```python
from build123d import *

# Parameters (mm, degrees)
F0_W          = 50.5
F0_H          = 50.5
F1_DEPTH      = 7.2
F2_W          = 45.2
F2_H          = 45.2
F3_DEPTH      = 5
F4_W          = 42
F4_H          = 42
F5_DEPTH      = 5
F5_DEPTH_BACK = 3
F6_R          = 2.5
F7_R          = 2
F8_SIZE       = 1
F9_R          = 1


with BuildPart() as f1:
    # F0 (on Top) → F1 (new body)
    with BuildSketch(Plane.XY):
        Rectangle(F0_W, F0_H)
    extrude(amount=F1_DEPTH)

    # F2 (on face) → F3 (join)
    with BuildSketch(Plane.XY.offset(7.2)):
        Rectangle(F2_W, F2_H)
    extrude(amount=F3_DEPTH)

    # F4 (on face) → F5 (cut, two sides)
    with BuildSketch(Plane.XY.offset(7.2)) as f5_sk:
        Rectangle(F4_W, F4_H)
    extrude(amount=F5_DEPTH, mode=Mode.SUBTRACT)
    extrude(f5_sk.sketch, amount=-F5_DEPTH_BACK, mode=Mode.SUBTRACT)

    # F6
    f6_edges = [f1.edges().sort_by_distance(p)[0] for p in [
        (-25.25, 25.25, 3.6),
        (-25.25, -25.25, 3.6),
        (25.25, -25.25, 3.6),
        (25.25, 25.25, 3.6),
        (-22.6, 22.6, 9.7),
        (-22.6, -22.6, 9.7),
        (22.6, -22.6, 9.7),
        (22.6, 22.6, 9.7),
    ]]
    fillet(f6_edges, radius=F6_R)

    # F7
    f7_edges = [f1.edges().sort_by_distance(p)[0] for p in [
        (-21, 21, 8.2),
        (21, 21, 8.2),
        (21, -21, 8.2),
        (-21, -21, 8.2),
    ]]
    fillet(f7_edges, radius=F7_R)

    # F8
    f8_edges = [f1.edges().sort_by_distance(p)[0] for p in [
        (-22.6, 0, 12.2),
    ]]
    chamfer(f8_edges, length=F8_SIZE)

    # F9
    f9_edges = [f1.edges().sort_by_distance(p)[0] for p in [
        (0, 25.25, 0),
    ]]
    fillet(f9_edges, radius=F9_R)


solid = f1.part
```
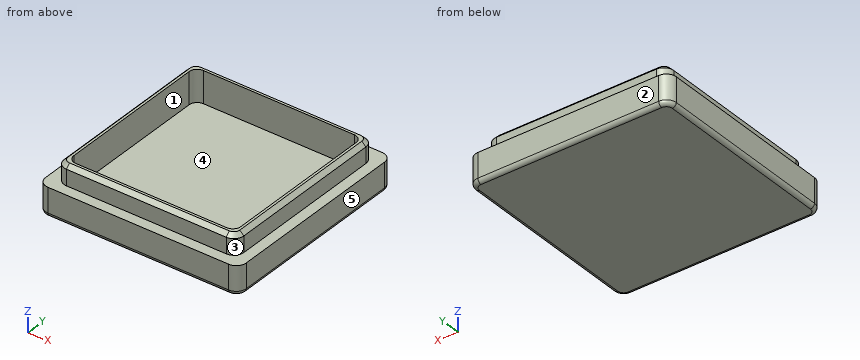
Verification items for the finished model (mm, model axes). Face numbers are marked on the shaded views. A direction names the side the tool comes from. Give positions to 0.01 mm unless a question says otherwise; leave off trailing zeros. Loops run counter-clockwise (first coordinate to the right, second up) from the corner with the lowest first, then second, coordinate; pieces in that order, holes last.
1. Go/stop test with flat-tipped pins: pin 1 Ø4 at (x, z) = (-3.5, 10) entering from -Y; pin 2 Ø8 at (x, y) = (-9, 1) entering from +Z; pin 3 Ø2.5 at (y, z) = (-9, 10) entering from +X. Record where each tip stops, or that it passes through.
2. Set-up check for the marked faces 1 and 2: record each of +Z, -Z, +X, -X, +Y, -Y from which the full face is reachable in a straight line by a thin tool's end or side.
3. Section check B-B, the plane y = -2. Enter the section's corners in (x, z), then the cut area to 3 significant figures.
4. Thickness scan on line 1 (X direction, y = 12, z = 10); line 2 (Y direction, x = 13, z = 5.5). Record the ranges inside material, lowest first.
5. Mould release check, pull along Y, two halves, no side actions. Record for the marked faces 3, 4 and 5: released by +Y, released by -Y, zero draft, split by the parting line, or undercut.
6. Section check A-A, the plane z = 8. Enter the section's corners in (x, y), then the cut area to 3 significant figures.
Geometry says:
1. pin 1: stops at y = -22.6
1. pin 2: stops at z = 4.2
1. pin 3: stops at x = 22.6
2. face 1: +Z
2. face 2: +Z, -Z, +X, -X, +Y
3. outline: (-25.25, 1) arc R1 ccw to (-24.25, 0) - (24.25, 0) arc R1 ccw to (25.25, 1) - (25.25, 7.2) - (22.6, 7.2) - (22.6, 11.2) - (21.6, 12.2) - (21, 12.2) - (21, 4.2) - (-21, 4.2) - (-21, 12.2) - (-21.6, 12.2) - (-22.6, 11.2) - (-22.6, 7.2) - (-25.25, 7.2) - close
3. area: 252 mm2
4. line 1: x = -22.6 to -21, 21 to 22.6
4. line 2: y = -25.25 to -21, 21 to 25.25
5. face 3: released by -Y
5. face 4: undercut
5. face 5: zero draft
6. outline: (-22.6, -20.1) arc R2.5 ccw to (-20.1, -22.6) - (20.1, -22.6) arc R2.5 ccw to (22.6, -20.1) - (22.6, 20.1) arc R2.5 ccw to (20.1, 22.6) - (-20.1, 22.6) arc R2.5 ccw to (-22.6, 20.1) - close; hole (-21, -19) arc R2 ccw to (-19, -21) - (19, -21) arc R2 ccw to (21, -19) - (21, 19) arc R2 ccw to (19, 21) - (-19, 21) arc R2 ccw to (-21, 19) - close
6. area: 277 mm2
